```python
from build123d import *

# Parameters (mm, degrees)
SKETCH1_W                        = 120
SKETCH1_H                        = 80
BOSS_EXTRUDE1_DEPTH              = 40
SKETCH2_R                        = 1.85
LINEAR_BEARING_SCREW_CUTS_DEPTH  = 14
SKETCH3_R                        = 9.5
LINEAR_BEARINGS_HOLE_DEPTH       = 55
SKETCH4_R                        = 1.875
LINEAR_BEARING_SCREW_CUTS2_DEPTH = 14
CUT_EXTRUDE4_START               = -55
SKETCH5_R                        = 9.5
CUT_EXTRUDE4_DEPTH               = 55
SKETCH11_R                       = 6
CUT_EXTRUDE9_DEPTH               = 111.566721937
SKETCH13_R                       = 2.5
CUT_EXTRUDE11_DEPTH              = 150.666295471


with BuildPart() as part:
    # Sketch1 → Boss-Extrude1 (new body)
    with BuildSketch(Plane.XY):
        with Locations((60, 40)):
            Rectangle(SKETCH1_W, SKETCH1_H)
    extrude(amount=BOSS_EXTRUDE1_DEPTH)

    # Sketch2 → linear-bearing-screw-cuts (cut)
    with BuildSketch(Plane.ZY):
        with Locations((30.25, 72.75)):
            Circle(SKETCH2_R)
        with Locations(Location((9.75, 72.75, 0), (0, 0, 180))):
            Circle(SKETCH2_R)
        with Locations(Location((30.25, 52.25, 0), (0, 0, 180))):
            Circle(SKETCH2_R)
        with Locations((9.75, 52.25)):
            Circle(SKETCH2_R)
        with Locations(Location((9.75, 27.75, 0), (0, 0, 180))):
            Circle(SKETCH2_R)
        with Locations((30.25, 27.75)):
            Circle(SKETCH2_R)
        with Locations(Location((30.25, 7.25, 0), (0, 0, 180))):
            Circle(SKETCH2_R)
        with Locations((9.75, 7.25)):
            Circle(SKETCH2_R)
    extrude(amount=-LINEAR_BEARING_SCREW_CUTS_DEPTH, mode=Mode.SUBTRACT)

    # Sketch3 → linear-bearings-hole (cut)
    with BuildSketch(Plane.ZY):
        with Locations((20, 62.5)):
            Circle(SKETCH3_R)
        with Locations(Location((20, 17.5, 0), (0, 0, 180))):
            Circle(SKETCH3_R)
    extrude(amount=-LINEAR_BEARINGS_HOLE_DEPTH, mode=Mode.SUBTRACT)

    # Sketch4 → linear-bearing-screw-cuts2 (cut)
    with BuildSketch(Plane(origin=(120, 0, 0), x_dir=(0, 0, -1), z_dir=(1, 0, 0))):
        with Locations((-9.75, 72.75)):
            Circle(SKETCH4_R)
        with Locations(Location((-30.25, 72.75, 0), (0, 0, 180))):
            Circle(SKETCH4_R)
        with Locations(Location((-9.75, 52.25, 0), (0, 0, 180))):
            Circle(SKETCH4_R)
        with Locations((-30.25, 52.25)):
            Circle(SKETCH4_R)
        with Locations(Location((-30.25, 27.75, 0), (0, 0, 180))):
            Circle(SKETCH4_R)
        with Locations((-9.75, 27.75)):
            Circle(SKETCH4_R)
        with Locations(Location((-9.75, 7.25, 0), (0, 0, 180))):
            Circle(SKETCH4_R)
        with Locations((-30.25, 7.25)):
            Circle(SKETCH4_R)
    extrude(amount=-LINEAR_BEARING_SCREW_CUTS2_DEPTH, mode=Mode.SUBTRACT)

    # Sketch5 → Cut-Extrude4 (cut)
    with BuildSketch(Plane(origin=(120, 0, 0), x_dir=(0, 0, -1), z_dir=(1, 0, 0)).offset(CUT_EXTRUDE4_START)):
        with Locations(Location((-20, 62.5, 0), (0, 0, 180))):
            Circle(SKETCH5_R)
        with Locations((-20, 17.5)):
            Circle(SKETCH5_R)
    extrude(amount=CUT_EXTRUDE4_DEPTH, mode=Mode.SUBTRACT)

    # Sketch11 → Cut-Extrude9 (cut, through all)
    with BuildSketch(Plane(origin=(65, 0, 0), x_dir=(0, 0, -1), z_dir=(1, 0, 0))):
        with Locations((-20, 62.5)):
            Circle(SKETCH11_R)
        with Locations((-20, 17.5)):
            Circle(SKETCH11_R)
    extrude(amount=-CUT_EXTRUDE9_DEPTH, mode=Mode.SUBTRACT)

    # Sketch13 → Cut-Extrude11 (cut, through all)
    with BuildSketch(Plane(origin=(0, 0, 0), x_dir=(-1, 0, 0), z_dir=(0, 0, -1))):
        with Locations((-102, 5)):
            Circle(SKETCH13_R)
        with Locations((-18, 5)):
            Circle(SKETCH13_R)
    extrude(amount=-CUT_EXTRUDE11_DEPTH, mode=Mode.SUBTRACT)


solid = part.part
```
Can you work these out from the model? Positions are in its coordinate system, mm. A direction names the side the tool comes from. Round coordinates to 2 decimals unless told otherwise and drop trailing zeros. Loops run counter-clockwise (first coordinate to the right, second up) from the corner with the lowest first, then second, coordinate; pieces in that order, holes last.
Item 1: Suppose I cut it at A-A, the plane x = 18. Write out the boundary of the cut face in (y, z).
Item 2: Please list where these lines run through material, in increasing order: L1, parallel to Y at x = 115.5, z = 9.75 (3 decimals); L2, parallel to Y at x = 80, z = 20; L3, parallel to Z at x = 4, y = 7.
Item 3: Will these pins go through, and if not, where does the flat tip stop? pin 1 Ø5.5 at (y, z) = (20, 17) entering from -X; pin 2 Ø2 at (y, z) = (7.25, 9.75) entering from +X.
Item 4: Which directions (+Z, -Z, +X, -X, +Y, -Y) give clear straight access to the entire face, cutting with the end or side of a thin tool? Please do faces 3 (the cylindrical face through (27.12, 71.92, 18.76)), 4 (the flat face through (65, 17.6, 13.8)).
Item 5: Suppose I cut it at D-D, the plane x = 38. Write out the boundary of the cut face in (y, z), then the cut area to 3 significant figures.
Item 6: Suppose I cut it at B-B, the plane z = 20. State how many separate pieces and enclosed holes the cut face has, then the cut area to 3 significant figures.
Item 7: If we mould it in two halves opening along Y, with no side actions, what happens to faces 1 (the flat face through (59, 80, 20)), 2 (the flat face through (55, 17.4, 13.8))? For each: +Y half, -Y half, draft (parallel to the pull), parting line (faces both ways), or undercut.
Item 8: Suppose I cut it at C-C, the plane y = 62.5. Write out the boundary of the cut face in (x, z), then the cut area to 3 significant figures.
Reported:
1. outline: (0, 0) - (2.5, 0) - (2.5, 40) - (0, 40) - close; (7.5, 0) - (80, 0) - (80, 40) - (7.5, 40) - close; hole circle Ø19 at (17.5, 20); hole circle Ø19 at (62.5, 20)
2. L1: y = 0 to 5.375, 9.125 to 25.875, 29.625 to 50.375, 54.125 to 70.875, 74.625 to 80
2. L2: y = 0 to 8, 27 to 53, 72 to 80
2. L3: z = 0 to 7.92, 11.58 to 28.42, 32.08 to 40
3. pin 1: stops at x = 55
3. pin 2: stops at x = 106
4. face 3: -X
4. face 4: +X
5. outline: (0, 0) - (80, 0) - (80, 40) - (0, 40) - close; hole circle Ø19 at (17.5, 20); hole circle Ø19 at (62.5, 20)
5. area: 2,630 mm2
6. separate pieces: 3
6. enclosed holes: 2
6. area: 5,140 mm2
7. face 1: +Y half
7. face 2: undercut
8. outline: (0, 0) - (120, 0) - (120, 10.5) - (65, 10.5) - (65, 14) - (55, 14) - (55, 10.5) - (0, 10.5) - close; (0, 29.5) - (55, 29.5) - (55, 26) - (65, 26) - (65, 29.5) - (120, 29.5) - (120, 40) - (0, 40) - close
8. area: 2,590 mm2
